```python
from build123d import *

# Parameters (mm, degrees)
ESQUISSE1_R                           = 2.25
ESQUISSE1_R_2                         = 4
ESQUISSE1_R_3                         = 1.6
T_LE_DE_BASE_PLI_E1_DEPTH             = 1.5
T_LE_PLI_E_SUR_AR_TE1_STRIP_W         = 9.81
T_LE_PLI_E_SUR_AR_TE1_STRIP_H         = 1.5
T_LE_PLI_E_SUR_AR_TE1_STRIP_CUT_DEPTH = 41.2
T_LE_PLI_E_SUR_AR_TE1_DEPTH           = 41.2
CONG_1_R                              = 3
ESQUISSE9_R                           = 1.6
ENL_V_MAT_EXTRU_1_DEPTH               = 10
T_LE_PLI_E_SUR_AR_TE2_STRIP_W         = 9.81
T_LE_PLI_E_SUR_AR_TE2_STRIP_H         = 1.5
T_LE_PLI_E_SUR_AR_TE2_STRIP_CUT_DEPTH = 8
T_LE_PLI_E_SUR_AR_TE2_DEPTH           = 8
T_LE_PLI_E_SUR_AR_TE3_STRIP_W         = 9.81
T_LE_PLI_E_SUR_AR_TE3_STRIP_H         = 1.5
T_LE_PLI_E_SUR_AR_TE3_STRIP_CUT_DEPTH = 8
T_LE_PLI_E_SUR_AR_TE3_DEPTH           = 8
CONG_2_R                              = 3
ESQUISSE16_R                          = 2.25
ENL_V_MAT_EXTRU_2_DEPTH               = 10


# Sheet-metal steps are written as plain solids
with BuildPart() as part:
    # Esquisse1 → Tôle de base pliée1 (new body)
    with BuildSketch(Plane.XY):
        with BuildLine():
            Line((52.684779063, 187.695605254), (52.684779063, 166.115117635))
            ThreePointArc((52.684779063, 166.115117635), (53.563458719, 163.993797291), (55.684779063, 163.115117635))
            Line((55.684779063, 163.115117635), (60.684779063, 163.115117635))
            Line((60.684779063, 163.115117635), (60.684779063, 158.115117635))
            Line((60.684779063, 158.115117635), (101.884779063, 158.115117635))
            Line((101.884779063, 158.115117635), (101.884779063, 163.115117635))
            Line((101.884779063, 163.115117635), (106.884779063, 163.115117635))
            ThreePointArc((106.884779063, 163.115117635), (109.006099406, 163.993797291), (109.884779063, 166.115117635))
            Line((109.884779063, 166.115117635), (109.884779063, 187.695605254))
            Line((109.884779063, 187.695605254), (109.884779063, 188.915117635))
            Line((109.884779063, 188.915117635), (101.884779063, 188.915117635))
            Line((101.884779063, 188.915117635), (101.884779063, 183.915117635))
            Line((101.884779063, 183.915117635), (98.684779063, 183.915117635))
            Line((98.684779063, 183.915117635), (98.684779063, 189.815117635))
            ThreePointArc((98.684779063, 189.815117635), (97.806099406, 191.936437979), (95.684779063, 192.815117635))
            Line((95.684779063, 192.815117635), (66.884779063, 192.815117635))
            ThreePointArc((66.884779063, 192.815117635), (64.763458719, 191.936437979), (63.884779063, 189.815117635))
            Line((63.884779063, 189.815117635), (63.884779063, 183.915117635))
            Line((63.884779063, 183.915117635), (60.684779063, 183.915117635))
            Line((60.684779063, 183.915117635), (60.684779063, 188.915117635))
            Line((60.684779063, 188.915117635), (52.684779063, 188.915117635))
            Line((52.684779063, 188.915117635), (52.684779063, 187.695605254))
        make_face()
        with Locations((57.034779063, 180.915117635)):
            Circle(ESQUISSE1_R, mode=Mode.SUBTRACT)
        with Locations((57.034779063, 171.115117635)):
            Circle(ESQUISSE1_R, mode=Mode.SUBTRACT)
        with Locations((72.934779063, 180.915117635)):
            Circle(ESQUISSE1_R_2, mode=Mode.SUBTRACT)
        with Locations((72.934779063, 189.265117635)):
            Circle(ESQUISSE1_R_3, mode=Mode.SUBTRACT)
        with Locations((72.934779063, 172.565117635)):
            Circle(ESQUISSE1_R_3, mode=Mode.SUBTRACT)
        with Locations(Location((89.634779063, 172.565117635, 0), (0, 0, 180))):
            Circle(ESQUISSE1_R_3, mode=Mode.SUBTRACT)
        with Locations(Location((89.634779063, 189.265117635, 0), (0, 0, 180))):
            Circle(ESQUISSE1_R_3, mode=Mode.SUBTRACT)
        with Locations(Location((89.634779063, 180.915117635, 0), (0, 0, 180))):
            Circle(ESQUISSE1_R_2, mode=Mode.SUBTRACT)
        with Locations(Location((105.534779063, 171.115117635, 0), (0, 0, 180))):
            Circle(ESQUISSE1_R, mode=Mode.SUBTRACT)
        with Locations(Location((105.534779063, 180.915117635, 0), (0, 0, 180))):
            Circle(ESQUISSE1_R, mode=Mode.SUBTRACT)
        with BuildLine():
            Line((63.334779063, 182.515117635), (65.834779063, 182.515117635))
            ThreePointArc((65.834779063, 182.515117635), (67.434779063, 180.915117635), (65.834779063, 179.315117635))
            Line((65.834779063, 179.315117635), (63.334779063, 179.315117635))
            ThreePointArc((63.334779063, 179.315117635), (61.734779063, 180.915117635), (63.334779063, 182.515117635))
        make_face(mode=Mode.SUBTRACT)
        with BuildLine():
            Line((82.534779063, 182.515117635), (80.034779063, 182.515117635))
            ThreePointArc((80.034779063, 182.515117635), (78.434779063, 180.915117635), (80.034779063, 179.315117635))
            Line((80.034779063, 179.315117635), (82.534779063, 179.315117635))
            ThreePointArc((82.534779063, 179.315117635), (84.134779063, 180.915117635), (82.534779063, 182.515117635))
        make_face(mode=Mode.SUBTRACT)
        with BuildLine():
            Line((99.234779063, 182.515117635), (96.734779063, 182.515117635))
            ThreePointArc((96.734779063, 182.515117635), (95.134779063, 180.915117635), (96.734779063, 179.315117635))
            Line((96.734779063, 179.315117635), (99.234779063, 179.315117635))
            ThreePointArc((99.234779063, 179.315117635), (100.834779063, 180.915117635), (99.234779063, 182.515117635))
        make_face(mode=Mode.SUBTRACT)
    extrude(amount=-T_LE_DE_BASE_PLI_E1_DEPTH)

    # Tôle pliée sur arête1 strip (across the edge) → Tôle pliée sur arête1 strip cut (cut)
    with BuildSketch(Plane(origin=(60.684779063, 158.115117635, 0), x_dir=(0, 1, 0), z_dir=(1, 0, 0))):
        with Locations((-1.5, -0.75)):
            Rectangle(T_LE_PLI_E_SUR_AR_TE1_STRIP_W, T_LE_PLI_E_SUR_AR_TE1_STRIP_H)
    extrude(amount=T_LE_PLI_E_SUR_AR_TE1_STRIP_CUT_DEPTH, mode=Mode.SUBTRACT)

    # Tôle pliée sur arête1 section (across the edge) → Tôle pliée sur arête1 (add)
    with BuildSketch(Plane(origin=(60.684779063, 158.115117635, 0), x_dir=(0, 1, 0), z_dir=(1, 0, 0))):
        with BuildLine():
            Line((0, 1.905), (0, 22.7))
            Line((0, 22.7), (1.5, 22.7))
            Line((1.5, 22.7), (1.5, 1.905))
            ThreePointArc((1.5, 1.905), (2.057961582, 0.557961582), (3.405, 0))
            Line((3.405, 0), (3.405, -1.5))
            ThreePointArc((3.405, -1.5), (0.99730141, -0.50269859), (0, 1.905))
        make_face()
    extrude(amount=T_LE_PLI_E_SUR_AR_TE1_DEPTH)

    # Congé1
    cong_1_edges = [part.edges().sort_by_distance(p)[0] for p in [
        (60.684779063, 158.865117635, 22.7),
        (101.884779063, 158.865117635, 22.7),
    ]]
    fillet(cong_1_edges, radius=CONG_1_R)

    # Esquisse9 → Enlèv. mat.-Extru.1 (cut)
    with BuildSketch(Plane(origin=(0, 159.615117635, 0), x_dir=(1, 0, 0), z_dir=(0, 1, 0))):
        with Locations(Location((71.334779063, -12.8, 0), (0, 0, 270))):
            Circle(ESQUISSE9_R)
        with Locations(Location((91.234779063, -12.8, 0), (0, 0, 270))):
            Circle(ESQUISSE9_R)
    extrude(amount=-ENL_V_MAT_EXTRU_1_DEPTH, mode=Mode.SUBTRACT)

    # Tôle pliée sur arête2 strip (across the edge) → Tôle pliée sur arête2 strip cut (cut)
    with BuildSketch(Plane(origin=(60.684779063, 188.915117635, 0), x_dir=(0, -1, 0), z_dir=(-1, 0, 0))):
        with Locations((-1.5, -0.75)):
            Rectangle(T_LE_PLI_E_SUR_AR_TE2_STRIP_W, T_LE_PLI_E_SUR_AR_TE2_STRIP_H)
    extrude(amount=T_LE_PLI_E_SUR_AR_TE2_STRIP_CUT_DEPTH, mode=Mode.SUBTRACT)

    # Tôle pliée sur arête2 section (across the edge) → Tôle pliée sur arête2 (add)
    with BuildSketch(Plane(origin=(60.684779063, 188.915117635, 0), x_dir=(0, -1, 0), z_dir=(-1, 0, 0))):
        with BuildLine():
            Line((0, 1.905), (0, 22.7))
            Line((0, 22.7), (1.5, 22.7))
            Line((1.5, 22.7), (1.5, 1.905))
            ThreePointArc((1.5, 1.905), (2.057961582, 0.557961582), (3.405, 0))
            Line((3.405, 0), (3.405, -1.5))
            ThreePointArc((3.405, -1.5), (0.99730141, -0.50269859), (0, 1.905))
        make_face()
    extrude(amount=T_LE_PLI_E_SUR_AR_TE2_DEPTH)

    # Tôle pliée sur arête3 strip (across the edge) → Tôle pliée sur arête3 strip cut (cut)
    with BuildSketch(Plane(origin=(109.884779063, 188.915117635, 0), x_dir=(0, -1, 0), z_dir=(-1, 0, 0))):
        with Locations((-1.5, -0.75)):
            Rectangle(T_LE_PLI_E_SUR_AR_TE3_STRIP_W, T_LE_PLI_E_SUR_AR_TE3_STRIP_H)
    extrude(amount=T_LE_PLI_E_SUR_AR_TE3_STRIP_CUT_DEPTH, mode=Mode.SUBTRACT)

    # Tôle pliée sur arête3 section (across the edge) → Tôle pliée sur arête3 (add)
    with BuildSketch(Plane(origin=(109.884779063, 188.915117635, 0), x_dir=(0, -1, 0), z_dir=(-1, 0, 0))):
        with BuildLine():
            Line((0, 1.905), (0, 22.7))
            Line((0, 22.7), (1.5, 22.7))
            Line((1.5, 22.7), (1.5, 1.905))
            ThreePointArc((1.5, 1.905), (2.057961582, 0.557961582), (3.405, 0))
            Line((3.405, 0), (3.405, -1.5))
            ThreePointArc((3.405, -1.5), (0.99730141, -0.50269859), (0, 1.905))
        make_face()
    extrude(amount=T_LE_PLI_E_SUR_AR_TE3_DEPTH)

    # Congé2
    cong_2_edges = [part.edges().sort_by_distance(p)[0] for p in [
        (60.684779063, 188.165117635, 22.7),
        (52.684779063, 188.165117635, 22.7),
        (109.884779063, 188.165117635, 22.7),
        (101.884779063, 188.165117635, 22.7),
    ]]
    fillet(cong_2_edges, radius=CONG_2_R)

    # Esquisse16 → Enlèv. mat.-Extru.2 (cut)
    with BuildSketch(Plane(origin=(0, 188.915117635, 0), x_dir=(1, 0, 0), z_dir=(0, 1, 0))):
        with Locations(Location((57.034779063, -7.8, 0), (0, 0, 270))):
            Circle(ESQUISSE16_R)
        with Locations(Location((57.034779063, -17.6, 0), (0, 0, 270))):
            Circle(ESQUISSE16_R)
        with Locations(Location((105.534779063, -7.8, 0), (0, 0, 270))):
            Circle(ESQUISSE16_R)
        with Locations(Location((105.534779063, -17.6, 0), (0, 0, 270))):
            Circle(ESQUISSE16_R)
    extrude(amount=-ENL_V_MAT_EXTRU_2_DEPTH, mode=Mode.SUBTRACT)


solid = part.part
```
Verification items for the finished model (mm, model axes). A direction names the side the tool comes from. Give positions to 0.01 mm unless a question says otherwise; leave off trailing zeros. Loops run counter-clockwise (first coordinate to the right, second up) from the corner with the lowest first, then second, coordinate; pieces in that order, holes last.
1. Section check D-D, the plane x = 87. Enter the section's corners in (y, z) (3 decimals), then the cut area to 3 significant figures.
2. Section check B-B, the plane x = 104. Enter the section's corners in (y, z) (3 decimals), then the cut area to 3 significant figures.
3. Thickness scan on line 1 (X direction, y = 159, z = 12.8); line 2 (X direction, y = 187.8, z = 17.6); line 3 (Z direction, x = 66.5, y = 161.5). Record the ranges inside material, lowest first.
4. Section check C-C, the plane y = 180. Count the separate pieces of the cut face and the enclosed holes in it, then the cut area to 3 significant figures.
5. Mould release check, pull along X, two halves, no side actions. Record for faces 1 (the cylindrical face through (105.94, 187.89, -0.53)), 2 (the cylindrical face through (53.54, 164.02, -0.74)), 3 (the cylindrical face through (71.665, 188.292, -0.74)), 4 (the cylindrical face through (72.07, 177.01, -0.74)): released by +X, released by -X, zero draft, split by the parting line, or undercut.
6. Go/stop test with flat-tipped pins: pin 1 Ø2.5 at (y, z) = (160, 5) entering from +X; pin 2 Ø7 at (x, y) = (57.03, 171.12) entering from -Z; pin 3 Ø3 at (x, y) = (92.5, 185.5) entering from +Z; pin 4 Ø4 at (y, z) = (161, 4) entering from -X. Record where each tip stops, or that it passes through.
7. Section check A-A, the plane z = 7.8. Enter the section's corners in (x, y).
8. Set-up check for faces 5 (the cylindrical face through (95.135, 180.95, -0.74)), 6 (the flat face through (106, 187.415, 12)), 7 (the flat face through (104, 163.115, -1)): record each of +Z, -Z, +X, -X, +Y, -Y from which the full face is reachable in a straight line by a thin tool's end or side.
Geometry says:
1. outline: (158.115, 1.905) arc R3.405 ccw to (161.52, -1.5) - (177.905, -1.5) - (177.905, 0) - (161.52, 0) arc R1.905 cw to (159.615, 1.905) - (159.615, 22.7) - (158.115, 22.7) - close; (183.925, -1.5) - (192.815, -1.5) - (192.815, 0) - (183.925, 0) - close
1. area: 75.4 mm2
2. outline: (163.115, -1.5) - (169.47, -1.5) - (169.47, 0) - (163.115, 0) - close; (172.76, -1.5) - (179.27, -1.5) - (179.27, 0) - (172.76, 0) - close; (182.56, -1.5) - (185.51, -1.5) arc R3.405 ccw to (188.915, 1.905) - (188.915, 6.155) - (187.415, 6.155) - (187.415, 1.905) arc R1.905 cw to (185.51, 0) - (182.56, 0) - close; (187.415, 9.445) - (188.915, 9.445) - (188.915, 15.955) - (187.415, 15.955) - close; (187.415, 19.245) - (188.915, 19.245) - (188.915, 22.567) - (187.415, 22.567) - close
2. area: 51.1 mm2
3. line 1: x = 60.68 to 69.73, 72.93 to 89.63, 92.83 to 101.88
3. line 2: x = 52.68 to 54.78, 59.28 to 60.68, 101.88 to 103.28, 107.78 to 109.88
3. line 3: z = -1.5 to 0
4. separate pieces: 8
4. enclosed holes: 0
4. area: 27.0 mm2
5. face 1: zero draft
5. face 2: released by -X
5. face 3: undercut
5. face 4: undercut
6. pin 1: stops at x = 101.88
6. pin 2: stops at z = -1.5
6. pin 3: stops at z = 0
6. pin 4: stops at x = 60.68
7. outline: (52.68, 187.42) - (54.78, 187.42) - (54.78, 188.92) - (52.68, 188.92) - close; (59.28, 187.42) - (60.68, 187.42) - (60.68, 188.92) - (59.28, 188.92) - close; (60.68, 158.12) - (101.88, 158.12) - (101.88, 159.62) - (60.68, 159.62) - close; (101.88, 187.42) - (103.28, 187.42) - (103.28, 188.92) - (101.88, 188.92) - close; (107.78, 187.42) - (109.88, 187.42) - (109.88, 188.92) - (107.78, 188.92) - close
8. face 5: +Z, -Z
8. face 6: +Z, +X, -X, -Y
8. face 7: +Z, -Z, +X, -Y
